Can you work these out from the model? Positions are in its coordinate system, mm. Coordinates: 2 decimals unless noted, no trailing zeros. Loops run counter-clockwise (first coordinate to the right, second up) from the corner with the lowest first, then second, coordinate; pieces in that order, holes last.
```python
from build123d import *

# Parameters (mm, degrees)
CROQUIS1_W              = 1001.972554514
CROQUIS1_H              = 550
SALIENTE_EXTRUIR1_DEPTH = 30
CROQUIS2_W              = 971.972554514
CROQUIS2_H              = 520
CORTAR_EXTRUIR1_DEPTH   = 2
REDONDEO1_R             = 8


with BuildPart() as part:
    # Croquis1 → Saliente-Extruir1 (new body)
    with BuildSketch(Plane.XY):
        with Locations((500.986277257, 275)):
            Rectangle(CROQUIS1_W, CROQUIS1_H)
    extrude(amount=SALIENTE_EXTRUIR1_DEPTH)

    # Croquis2 → Cortar-Extruir1 (cut)
    with BuildSketch(Plane.XY.offset(30)):
        with Locations((500.986277257, 275)):
            Rectangle(CROQUIS2_W, CROQUIS2_H)
    extrude(amount=-CORTAR_EXTRUIR1_DEPTH, mode=Mode.SUBTRACT)

    # Redondeo1
    redondeo1_edges = [part.edges().sort_by_distance(p)[0] for p in [
        (0, 550, 15),
        (1001.972554514, 550, 15),
        (1001.972554514, 0, 15),
        (0, 0, 15),
    ]]
    fillet(redondeo1_edges, radius=REDONDEO1_R)


solid = part.part
```
(1) If we mould it in two halves opening along Y, with no side actions, what happens to faces 1 (the flat face through (494, 279, 28)), 2 (the flat face through (494, 550, 15)), 3 (the flat face through (494, 279, 0)), 4 (the flat face through (494, 0, 15))? For each: released by +Y, released by -Y, zero draft, split by the parting line, or undercut.
Check values:
face 1: undercut
face 2: released by +Y
face 3: zero draft
face 4: released by -Y
(2) If I drill on probe 1 along Z at (x, y) = (301, 59), over which ranges is the centre line in solid material (lowest first)?
Check values:
probe 1: z = 0 to 28
(3) I want a section at A-A on y = 110.5. Write out the boundary of the cut face in (x, z), then the cut area to 3 significant figures.
Check values:
outline: (0, 0) - (1001.97, 0) - (1001.97, 30) - (986.97, 30) - (986.97, 28) - (15, 28) - (15, 30) - (0, 30) - close
area: 28,100 mm2
(4) I want a section at B-B on x = 600. Write out the boundary of the cut face in (y, z), then the cut area to 3 significant figures.
Check values:
outline: (0, 0) - (550, 0) - (550, 30) - (535, 30) - (535, 28) - (15, 28) - (15, 30) - (0, 30) - close
area: 15,500 mm2
(5) I'm going to push a flat-ended pin straight in: pin 1 (3 mm diameter, centred on x = 103, y = 373, fed in from +Z). Where does the tip first touch, or does it pass through?
Check values:
pin 1: stops at z = 28
